```python
from build123d import *

# Parameters (mm, degrees)
SKETCH_1_W          = 30
SKETCH_1_H          = 37.5
EXTRUDE_2_DEPTH     = 15
SKETCH_3_W          = 4.5
SKETCH_3_H          = 31.058772458
SKETCH_3_W_2        = 4.938881881
SKETCH_3_H_2        = 33
SKETCH_3_W_3        = 4.061118119
CUT_EXTRUDE_1_DEPTH = 51.311529494
SKETCH_4_R          = 7.5
CUT_EXTRUDE_2_DEPTH = 55.169268422
CHAMFER_1_SIZE      = 2


with BuildPart() as part:
    # 草图1 → 凸台-拉伸2 (new, symmetric)
    with BuildSketch(Plane(origin=(0, 0, 0), x_dir=(0, 0, -1), z_dir=(1, 0, 0))):
        with Locations((15, 18.75)):
            Rectangle(SKETCH_1_W, SKETCH_1_H)
    extrude(amount=EXTRUDE_2_DEPTH, both=True)

    # 草图3 → 切除-拉伸1 (cut, through all)
    with BuildSketch(Plane.XY):
        with Locations((-1.811118119, 21.970613771)):
            Rectangle(SKETCH_3_W, SKETCH_3_H)
        with Locations((2.688881881, 21.970613771)):
            Rectangle(SKETCH_3_W, SKETCH_3_H)
        with Locations((-12.53055906, 21)):
            Rectangle(SKETCH_3_W_2, SKETCH_3_H_2)
        with Locations((12.969440941, 21)):
            Rectangle(SKETCH_3_W_3, SKETCH_3_H_2)
    extrude(amount=-CUT_EXTRUDE_1_DEPTH, mode=Mode.SUBTRACT)

    # 草图4 → 切除-拉伸2 (cut, through all)
    with BuildSketch(Plane.ZY.offset(10.061118119)):
        with Locations((-15, 25.5)):
            Circle(SKETCH_4_R)
    extrude(amount=-CUT_EXTRUDE_2_DEPTH, mode=Mode.SUBTRACT)

    # 倒角1
    chamfer_1_edges = [part.edges().sort_by_distance(p)[0] for p in [
        (15, 2.25, -30),
        (-15, 2.25, 0),
        (15, 2.25, 0),
        (7.938881881, 37.5, 0),
        (-7.061118119, 37.5, 0),
        (7.938881881, 37.5, -30),
        (-7.061118119, 37.5, -30),
        (-15, 2.25, -30),
    ]]
    chamfer(chamfer_1_edges, length=CHAMFER_1_SIZE)


solid = part.part
```
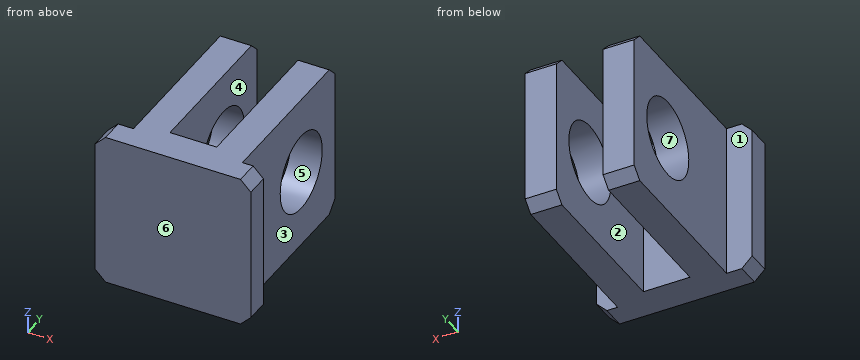
Source: CAD feature listing. Evaluate the final solid. Frame: model axes, mm. Face numbers are marked on the shaded views. A direction names the side the tool comes from. Give positions to 0.01 mm unless a question says otherwise; leave off trailing zeros. Loops run counter-clockwise (first coordinate to the right, second up) from the corner with the lowest first, then second, coordinate; pieces in that order, holes last. Notation, with made-up numbers: (17, 31) -> (47, 31) arc R14 cw to (47, 45) -> close; hole circle Ø2 at (4.25, 28.25). An arc over 180 degrees is marked (long way). Put each result on its own line as item: value. Start each with the question number.
1) Cut plane D-D (z = -25). Return loops of the section in (x, y).
2) Material intervals for probe 1 along X at (y, z) = (25.5, -3.25); probe 2 along Y at (x, z) = (-5.65, -15); probe 3 along Y at (x, z) = (3.5, -3.25), sorted ascending.
3) Cut plane A-A (y = 25.5). Return loops of the section in (x, z), then the cut area to 3 significant figures.
4) Cut plane C-C (x = 8). Return loops of the section in (y, z).
5) Reachability of the marked faces 1, 2 and 3 from +Z, -Z, +X, -X, +Y, -Y: full face, straight path, thin tool, end or side. Return the list, or none.
6) Cut plane B-B (z = -15). Return loops of the section in (x, y).
7) Draft query along Y for the marked faces 4, 5, 6 and 7. Return one class per face: released by +Y, released by -Y, zero draft, split by the parting line, or undercut.
8) Contact query for flat-ended pins moving along their axis: P1, Ø10, axis at x = -10.5, y = 31.5, coming from the -Z side; P2, Ø7, axis at x = 0.5, z = -17, coming from the +Y side; P3, Ø10, axis at y = 10, z = -10, coming from the +X side; P4, Ø5.5, axis at x = -13, z = -12, coming from the +Y side. Output: stop coordinate, or through.
Results are:
1. outline: (-15, 0) -> (15, 0) -> (15, 4.5) -> (10.94, 4.5) -> (10.94, 37.5) -> (4.94, 37.5) -> (4.94, 6.44) -> (-4.06, 6.44) -> (-4.06, 37.5) -> (-10.06, 37.5) -> (-10.06, 4.5) -> (-15, 4.5) -> close
2. probe 1: x = -10.06 to -4.06, 4.94 to 10.94
2. probe 2: y = 0 to 18, 33 to 37.5
2. probe 3: y = 0 to 6.44
3. outline: (-10.06, -30) -> (-4.06, -30) -> (-4.06, -22.5) -> (-10.06, -22.5) -> close; (-10.06, -7.5) -> (-4.06, -7.5) -> (-4.06, 0) -> (-10.06, 0) -> close; (4.94, -30) -> (10.94, -30) -> (10.94, -22.5) -> (4.94, -22.5) -> close; (4.94, -7.5) -> (10.94, -7.5) -> (10.94, 0) -> (4.94, 0) -> close
3. area: 180 mm2
4. outline: (0, -30) -> (35.5, -30) -> (37.5, -28) -> (37.5, -2) -> (35.5, 0) -> (0, 0) -> close; hole circle Ø15 at (25.5, -15)
5. face 1: +Z, -Z, -X, +Y
5. face 2: +Z, -Z, +Y
5. face 3: +Z, -Z, +X, +Y
6. outline: (-15, 0) -> (15, 0) -> (15, 4.5) -> (10.94, 4.5) -> (10.94, 18) -> (4.94, 18) -> (4.94, 6.44) -> (-4.06, 6.44) -> (-4.06, 18) -> (-10.06, 18) -> (-10.06, 4.5) -> (-15, 4.5) -> close; (-10.06, 33) -> (-4.06, 33) -> (-4.06, 37.5) -> (-10.06, 37.5) -> close; (4.94, 33) -> (10.94, 33) -> (10.94, 37.5) -> (4.94, 37.5) -> close
7. face 4: zero draft
7. face 5: undercut
7. face 6: released by -Y
7. face 7: undercut
8. P1: stops at z = -30
8. P2: stops at y = 6.44
8. P3: stops at x = 10.94
8. P4: stops at y = 4.5
